Check sheet for the drawn part. Datum: minimum x, y, z corner. Units: mm. Round coordinates to 2 decimals unless told otherwise and drop trailing zeros. Write each loop counter-clockwise with the first axis right and the second up, starting at its lowest first coordinate (ties: lowest second). Pieces come first, ordered by that corner, then holes. Notation, with made-up numbers: (-12.75, 3.5) -> (-1.75, 3.5) arc R16 cw to (-1.75, 31.5) -> close; hole circle Ø8 at (-17.75, 14.25). An arc over 180 degrees is marked (long way). Use CSV: the item, a comma, the result in double quotes.
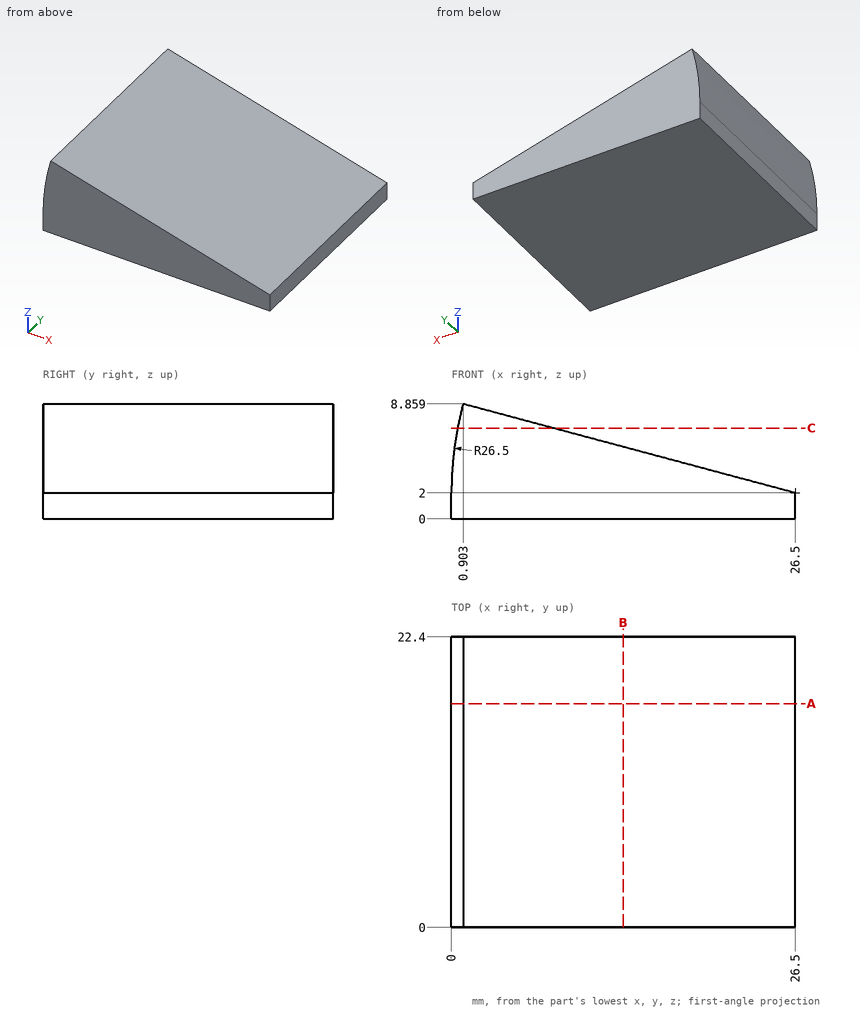
Q1. Section check A-A (y = 17.25). Record the cut outline in (x, z).
Filled in:
outline,"(0, 0) -> (26.5, 0) -> (26.5, 2) -> (0.9, 8.86) arc R26.5 ccw to (0, 2) -> close"
Q2. Section check B-B (x = 13.25). Record the cut outline in (y, z), plus the area to 3 significant figures.
Filled in:
outline,"(0, 0) -> (22.4, 0) -> (22.4, 5.55) -> (0, 5.55) -> close"
area,"124 mm²"
Q3. Section check C-C (z = 7). Record the cut outline in (x, y).
Filled in:
outline,"(0.48, 0) -> (7.84, 0) -> (7.84, 22.4) -> (0.48, 22.4) -> close"
Q4. Go/stop test with flat-tipped pins: P1, Ø10, axis at x = 18.5, y = 13.5, coming from the +Z side; P2, Ø5, axis at x = 20.5, y = 10.5, coming from the +Z side; P3, Ø4, axis at y = 2.5, z = 5.5, coming from the -X side. Record where each tip stops, or that it passes through.
Filled in:
P1,"z = 5.48"
P2,"z = 4.28"
P3,"x = 0.04"
Q5. Material ranges on L1, parallel to Z at x = 20.5, y = 12.25; L2, parallel to Z at x = 24.5, y = 11.5 (1 decimal), recorded low to high.
Filled in:
L1,"0 to 3.61"
L2,"0 to 2.5"
